```python
from build123d import *

# Parameters (mm, degrees)
SKETCH049_W     = 17
SKETCH049_H     = 7.6
PAD022_DEPTH    = 0.8
SKETCH050_W     = 3
SKETCH050_H     = 3.6
PAD023_DEPTH    = 3
SKETCH051_W     = 4
SKETCH051_H     = 1.6
POCKET017_DEPTH = 0.801


with BuildPart() as part:
    # Sketch049 → Pad022 (new body)
    with BuildSketch(Plane.YZ):
        Rectangle(SKETCH049_W, SKETCH049_H)
    extrude(amount=PAD022_DEPTH)

    # Sketch050 (on Face6 of Pad022) → Pad023 (join)
    with BuildSketch(Plane.YZ.offset(0.8)):
        with Locations((-6, 2)):
            Rectangle(SKETCH050_W, SKETCH050_H)
        with Locations((6, 2)):
            Rectangle(SKETCH050_W, SKETCH050_H)
    extrude(amount=PAD023_DEPTH)

    # Sketch051 (on Face5 of Pad023) → Pocket017 (cut, through all)
    with BuildSketch(Plane.YZ.offset(0.8)):
        with Locations((0, 1.8)):
            Rectangle(SKETCH051_W, SKETCH051_H)
    extrude(amount=-POCKET017_DEPTH, mode=Mode.SUBTRACT)


with BuildPart() as part_1:
    # Body006 placement: moved
    add(part.part.moved(Location((55.8, 12.5, 14))))


solid = part_1.part
```
The model under review builds one solid part; all positions refer to its coordinate system, in mm. A direction names the side the tool comes from. Give positions to 0.01 mm unless a question says otherwise; leave off trailing zeros. Write each loop counter-clockwise with the first axis right and the second up, starting at its lowest first coordinate (ties: lowest second). Pieces come first, ordered by that corner, then holes. Notation, with made-up numbers: (77.25, -34.5) - (113.25, -34.5) arc R16 ccw to (113.25, -18.5) - close; hole circle Ø6 at (-11, -11.5). An arc over 180 degrees is marked (long way). Answer in a Markdown table with one row per item. Add a question column.
1. We need section A-A on z = 15.5. Write out the cut boundary in (x, y).
2. We need section C-C on y = 11.25. Write out the cut boundary in (x, z).
3. We need section D-D on x = 56.15. Write out the cut boundary in (y, z), then the cut area to 3 significant figures.
4. Insertion check: P1, Ø0.9, axis at x = 58, z = 16, coming from the -Y side; P2, Ø1.5, axis at x = 58, y = 6, coming from the -Z side; P3, Ø1.5, axis at x = 58, z = 16.5, coming from the +Y side. Each pin has a flat end and moves straight along its axis. Give the tip position at first contact, or say it passes through.
5. We need section B-B on x = 59.1. Write out the cut boundary in (y, z).
6. Tool access review of faces 1 (the flat face through (58, 18, 14.2)), 2 (the flat face through (58, 17, 16)), 3 (the flat face through (59.6, 6, 16)), 4 (the flat face through (58, 20, 16)), 5 (the flat face through (55.8, 12, 14)): name each direction out of +Z, -Z, +X, -X, +Y, -Y from which nothing blocks a thin tool from reaching the whole face with its end or side.
7. Wall thickness on line 1 along Y through (x, z) = (56.9, 16.5); line 2 along Z through (x, y) = (57.9, 7.5); line 3 along Z through (x, y) = (56.15, 11.75): over which ranges is each line inside the solid? List them lowest first. Write a range as [from, to].
8. Draft analysis for pull direction Y (two halves, no side actions). For faces 6 (the flat face through (59.6, 18, 16)), 7 (the flat face through (58, 5, 16)), 8 (the flat face through (56.6, 12, 13)), 9 (the flat face through (58, 8, 16)), state which applies: +Y half, -Y half, draft (parallel to the pull), parting line (faces both ways), or undercut.
Ans:
| question | item | result |
|---|---|---|
| 1 | outline | (55.8, 4) - (56.6, 4) - (56.6, 5) - (59.6, 5) - (59.6, 8) - (56.6, 8) - (56.6, 10.5) - (55.8, 10.5) - close; (55.8, 14.5) - (56.6, 14.5) - (56.6, 17) - (59.6, 17) - (59.6, 20) - (56.6, 20) - (56.6, 21) - (55.8, 21) - close |
| 2 | outline | (55.8, 10.2) - (56.6, 10.2) - (56.6, 15) - (55.8, 15) - close; (55.8, 16.6) - (56.6, 16.6) - (56.6, 17.8) - (55.8, 17.8) - close |
| 3 | outline | (4, 10.2) - (21, 10.2) - (21, 17.8) - (4, 17.8) - close; hole (10.5, 15) - (14.5, 15) - (14.5, 16.6) - (10.5, 16.6) - close |
| 3 | area | 123 mm^2 |
| 4 | P1 | stops at y = 5 |
| 4 | P2 | stops at z = 14.2 |
| 4 | P3 | stops at y = 20 |
| 5 | outline | (5, 14.2) - (8, 14.2) - (8, 17.8) - (5, 17.8) - close; (17, 14.2) - (20, 14.2) - (20, 17.8) - (17, 17.8) - close |
| 6 | face 1 | -Z, +X, +Y, -Y |
| 6 | face 2 | +Z, -Z, +X |
| 6 | face 3 | +Z, -Z, +X, +Y, -Y |
| 6 | face 4 | +Z, -Z, +X, +Y |
| 6 | face 5 | +Z, -Z, -X, +Y, -Y |
| 7 | line 1 | y = [5, 8], [17, 20] |
| 7 | line 2 | z = [14.2, 17.8] |
| 7 | line 3 | z = [10.2, 15], [16.6, 17.8] |
| 8 | face 6 | draft |
| 8 | face 7 | -Y half |
| 8 | face 8 | undercut |
| 8 | face 9 | undercut |
